```python
from build123d import *

# Parameters (mm, degrees)
SKETCH1_R                = 6.35
BOSS_EXTRUDE1_DEPTH      = 57.15
BOSS_EXTRUDE2_DEPTH      = 187.5
BOSS_EXTRUDE2_DEPTH_BACK = 62.5
SKETCH2_R                = 6.35
BOSS_EXTRUDE3_START      = 47.625
SKETCH3_R                = 3.5
BOSS_EXTRUDE3_DEPTH      = 66.675


with BuildPart() as part:
    # Sketch1 → Boss-Extrude1 (new body)
    with BuildSketch(Plane(origin=(0, 0, 0), x_dir=(1, 0, 0), z_dir=(0, 1, 0))):
        with Locations(Location((0, 0, 0), (0, 0, 270))):
            Circle(SKETCH1_R)
    extrude(amount=BOSS_EXTRUDE1_DEPTH)

    # Sketch2 → Boss-Extrude2 (add, two sides: drawn at the far end of the back side and taken through both)
    with BuildSketch(Plane.XY.offset(-BOSS_EXTRUDE2_DEPTH_BACK)):
        with Locations((0, 57.15)):
            Circle(SKETCH2_R)
    extrude(amount=BOSS_EXTRUDE2_DEPTH + BOSS_EXTRUDE2_DEPTH_BACK)

    # Sketch3 → Boss-Extrude3 (add)
    with BuildSketch(Plane(origin=(0, 0, 0), x_dir=(1, 0, 0), z_dir=(0, 1, 0)).offset(BOSS_EXTRUDE3_START)):
        with Locations(Location((0, 14.875, 0), (0, 0, 90))):
            Circle(SKETCH3_R)
        with Locations(Location((0, 43.45, 0), (0, 0, 90))):
            Circle(SKETCH3_R)
    extrude(amount=BOSS_EXTRUDE3_DEPTH)


solid = part.part
```
Check sheet for the modelled part. Datum: model origin and axes. Units: mm. A direction names the side the tool comes from. Give positions to 0.01 mm unless a question says otherwise; leave off trailing zeros. Write each loop counter-clockwise with the first axis right and the second up, starting at its lowest first coordinate (ties: lowest second). Pieces come first, ordered by that corner, then holes.
Item 1: Cross-section at D-D (y = 35). Enter the section's corners in (x, z), and give its area (3 significant figures).
Item 2: Draft check along Z on faces 5 (the face through (0, 57, -62.5)), 6 (the face through (0, 0, 0)), 7 (the face through (-1.051, 88.011, -18.213)). Enter one of: released by +Z, released by -Z, zero draft, split by the parting line, or undercut.
Item 3: Scan lines: L1, parallel to Y at x = 0.75, z = 102.5; L2, parallel to Z at x = 0, y = 25; L3, parallel to Z at x = -2.5, y = 65.5. Record each from-to range of solid material in increasing order.
Item 4: Access from +Z, -Z, +X, -X, +Y, -Y to the whole of each face (thin tool, end or side, straight path). Record for faces 1 (the face through (1.907, 28.175, 6.057)), 2 (the face through (-0.827, 63.446, 60.75)), 3 (the face through (-1.05, 88.01, -46.79)), 4 (the face through (0, 47.625, -15)).
Item 5: Cross-section at C-C (z = 130). Enter the section's corners in (x, y), and give its area (3 significant figures).
Item 6: Gauge pin test, flat ends, axial feed: pin 1 (1 mm diameter, centred on x = -3, z = 58, fed in from +Y); pin 2 (1 mm diameter, centred on x = 1.5, y = 92, fed in from -Z); pin 3 (3.5 mm diameter, centred on x = -0.5, z = -44, fed in from -Y) (3 decimals). Record the tip position at first contact, or that the pin passes through.
Item 7: Cross-section at A-A (y = 87). Enter the section's corners in (x, z) (3 decimals), and give its area (3 significant figures).
Item 8: Cross-section at B-B (x = 0). Enter the section's corners in (y, z) (3 decimals), and give its area (3 significant figures).
Report:
1. outline: circle Ø12.7 at (0, 0)
1. area: 127 mm2
2. face 5: released by -Z
2. face 6: zero draft
2. face 7: undercut
3. L1: y = 50.84 to 63.46
3. L2: z = -6.35 to 6.35
3. L3: z = -45.9 to -41, -17.32 to -12.43
4. face 1: -Y
4. face 2: none
4. face 3: +Y
4. face 4: -Z, +X, -X, -Y
5. outline: circle Ø12.7 at (0, 57.15)
5. area: 127 mm2
6. pin 1: stops at y = 62.99
6. pin 2: stops at z = -46.8
6. pin 3: stops at y = 47.625
7. outline: circle Ø7 at (0, -43.45); circle Ø7 at (0, -14.875)
7. area: 77.0 mm2
8. outline: (0, -6.35) - (50.8, -6.35) - (50.8, -11.375) - (47.625, -11.375) - (47.625, -18.375) - (50.8, -18.375) - (50.8, -39.95) - (47.625, -39.95) - (47.625, -46.95) - (50.8, -46.95) - (50.8, -62.5) - (63.5, -62.5) - (63.5, -46.95) - (114.3, -46.95) - (114.3, -39.95) - (63.5, -39.95) - (63.5, -18.375) - (114.3, -18.375) - (114.3, -11.375) - (63.5, -11.375) - (63.5, 187.5) - (50.8, 187.5) - (50.8, 6.35) - (0, 6.35) - close
8. area: 4,580 mm2
